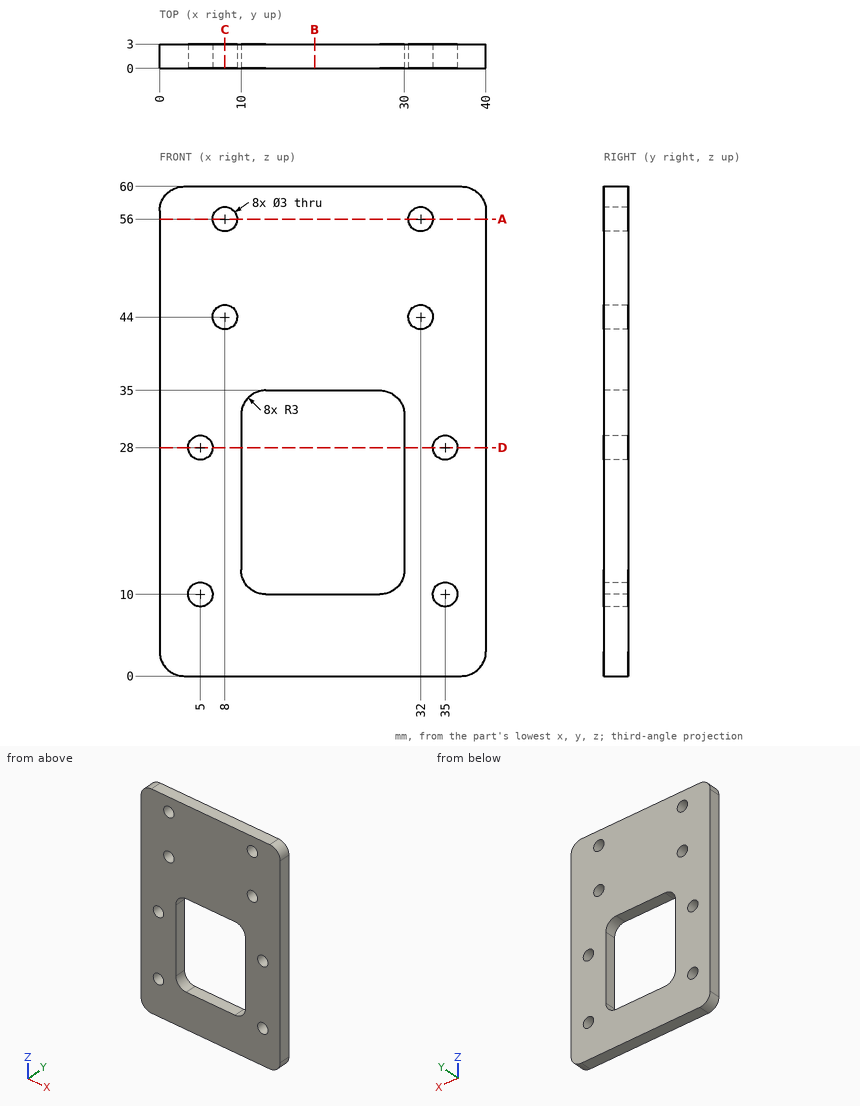
Geometry: see drawing. Coordinates: mm, zero at the bounding-box minimum. Coordinates: 2 decimals unless noted, no trailing zeros. Order: outer loops, then holes, each group sorted by start corner. A loop starts at its lowest first (then second) coordinate and runs counter-clockwise, first axis right, second up. Notation, with made-up numbers: M -18,12 L -6,12 A31 ccw -6,46 Z; hole C 22.25,78.5 d2. An arc over 180 degrees is marked long. Answer in a Markdown table with one row per item. Add a question column.
Q1. Section query B-B on x = 19. Return the cut outline in (y, z), and give its area (3 significant figures).
Q2. Section query A-A on z = 56. Return the cut outline in (x, y), and give its area (3 significant figures).
Q3. Contact query for flat-ended pins moving along their axis: P1, Ø5, axis at x = 5, z = 10, coming from the +Y side; P2, Ø1.8, axis at x = 32, z = 44, coming from the +Y side. Output: stop coordinate, or through.
Q4. Line query: L1, parallel to X at y = 2.2, z = 28; L2, parallel to X at y = 1.3, z = 56; L3, parallel to X at y = 2.85, z = 24.5. Output: solid intervals per line, ascending.
Q5. Section query C-C on x = 8. Return the cut outline in (y, z), and give its area (3 significant figures).
Q6. Section query D-D on z = 28. Return the cut outline in (x, y).
Completed:
| question | item | result |
|---|---|---|
| 1 | outline | M 0,0 L 3,0 L 3,10 L 0,10 Z; M 0,35 L 3,35 L 3,60 L 0,60 Z |
| 1 | area | 105 mm2 |
| 2 | outline | M 0,0 L 6.5,0 L 6.5,3 L 0,3 Z; M 9.5,0 L 30.5,0 L 30.5,3 L 9.5,3 Z; M 33.5,0 L 40,0 L 40,3 L 33.5,3 Z |
| 2 | area | 102 mm2 |
| 3 | P1 | stops at y = 3 |
| 3 | P2 | passes through |
| 4 | L1 | x = 0 to 3.5, 6.5 to 10, 30 to 33.5, 36.5 to 40 |
| 4 | L2 | x = 0 to 6.5, 9.5 to 30.5, 33.5 to 40 |
| 4 | L3 | x = 0 to 10, 30 to 40 |
| 5 | outline | M 0,0 L 3,0 L 3,42.5 L 0,42.5 Z; M 0,45.5 L 3,45.5 L 3,54.5 L 0,54.5 Z; M 0,57.5 L 3,57.5 L 3,60 L 0,60 Z |
| 5 | area | 162 mm2 |
| 6 | outline | M 0,0 L 3.5,0 L 3.5,3 L 0,3 Z; M 6.5,0 L 10,0 L 10,3 L 6.5,3 Z; M 30,0 L 33.5,0 L 33.5,3 L 30,3 Z; M 36.5,0 L 40,0 L 40,3 L 36.5,3 Z |
